Input: part model. Units: mm. Frame: model coordinates. Face numbers are marked on the shaded views. A direction names the side the tool comes from. Give positions to 0.01 mm unless a question says otherwise; leave off trailing zeros. Order: outer loops, then holes, each group sorted by start corner. A loop starts at its lowest first (then second) coordinate and runs counter-clockwise, first axis right, second up. Notation, with made-up numbers: (49.5, -29.75) -> (92.5, -29.75) arc R31 cw to (92.5, 2.25) -> close; hole circle Ø11 at (42, 18.25). An arc over 180 degrees is marked (long way). Use a Markdown table: item, result. Add a question column.
from build123d import *

# Parameters (mm, degrees)
EXTRUDE_1_DEPTH      = 25
CUT_EXTRUDE_4_DEPTH  = 80.457942189
SKETCH_7_W           = 16.60831278
SKETCH_7_H           = 38.473598513
CUT_EXTRUDE_14_DEPTH = 80.457942189
SKETCH_8_W           = 5
SKETCH_8_H           = 30.968526609
EXTRUDE_2_DEPTH      = 25
EXTRUDE_3_DEPTH      = 25
FILLET_2_R           = 3
FILLET_4_R           = 1
SKETCH_10_W          = 2
SKETCH_10_H          = 4
CUT_EXTRUDE_15_DEPTH = 78.792556685
SKETCH_11_W          = 10.357145721
SKETCH_11_H          = 16.019748685
CUT_EXTRUDE_16_DEPTH = 80.457942189


with BuildPart() as part:
    # Эскиз1 → Бобышка-Вытянуть1 (new body)
    with BuildSketch(Plane(origin=(0, 0, 0), x_dir=(1, 0, 0), z_dir=(0, 1, 0))):
        Polygon((-66.825757576, 34.969739794), (-66.825757576, 29.969739794), (-63.825757576, 29.969739794), (-63.825757576, 31.969739794), (-38.825757576, 31.969739794), (-38.825757576, 6.969739794), (-63.825757576, 6.969739794), (-63.825757576, 8.969739794), (-66.825757576, 8.969739794), (-66.825757576, 3.969739794), (-22.123470102, 3.969739794), (-36.579007505, 34.969739794), align=None)
    extrude(amount=EXTRUDE_1_DEPTH)

    # Эскиз3 → Вырез-Вытянуть4 (cut, through all)
    with BuildSketch(Plane.XZ):
        Polygon((-66.825757576, -3.969739794), (-65.325757576, -8.969739794), (-66.825757576, -8.969739794), align=None)
        Polygon((-66.825757576, -29.969739794), (-66.825757576, -34.969739794), (-65.325757576, -29.969739794), align=None)
    extrude(amount=-CUT_EXTRUDE_4_DEPTH, mode=Mode.SUBTRACT)

    # Эскиз7 → Вырез-Вытянуть14 (cut, through all)
    with BuildSketch(Plane(origin=(0, 0, 0), x_dir=(-1, 0, 0), z_dir=(0, -1, 0))):
        with Locations((27.703474463, 20.539743139)):
            Rectangle(SKETCH_7_W, SKETCH_7_H)
    extrude(amount=-CUT_EXTRUDE_14_DEPTH, mode=Mode.SUBTRACT)

    # Эскиз8 → Бобышка-Вытянуть2 (add)
    with BuildSketch(Plane(origin=(0, 0, 0), x_dir=(-1, 0, 0), z_dir=(0, -1, 0))):
        with Locations((36.298943925, 19.454003098)):
            Rectangle(SKETCH_8_W, SKETCH_8_H)
    extrude(amount=-EXTRUDE_2_DEPTH)

    # Эскиз9 → Бобышка-Вытянуть3 (add)
    with BuildSketch(Plane.XZ):
        with BuildLine():
            Line((-25.798943925, -9.121669553), (-24.000865345, -7.695483003))
            ThreePointArc((-24.000865345, -7.695483003), (-36.096342696, -11.954003099), (-24.000865345, -16.212523195))
            Line((-24.000865345, -16.212523195), (-25.798943925, -14.786336644))
            ThreePointArc((-25.798943925, -14.786336644), (-33.80140029, -11.954003099), (-25.798943925, -9.121669553))
        make_face()
        with BuildLine():
            Line((-25.798943925, -24.130682885), (-24.000865345, -22.7126007))
            ThreePointArc((-24.000865345, -22.7126007), (-36.0856317, -26.954003099), (-24.000865345, -31.195405497))
            Line((-24.000865345, -31.195405497), (-25.798943925, -29.777323313))
            ThreePointArc((-25.798943925, -29.777323313), (-33.795735785, -26.954003099), (-25.798943925, -24.130682885))
        make_face()
    extrude(amount=-EXTRUDE_3_DEPTH)

    # Скругление2
    # the kernel refuses this fillet: 3 mm, written as the material it adds along each edge
    with BuildSketch(Plane(origin=(-33.798943925, 25, -6.859434417), x_dir=(0, 0, 1), z_dir=(0, -1, 0))) as fillet_2_piece_1:
        with BuildLine():
            CenterArc((4.502629254, -2.529514158), FILLET_2_R, 122.523458888, 69.079199353)
            Line((1.563931496, -3.132884263), (1.505157541, -3.144951665))
            ThreePointArc((1.505157541, -3.144951665), (0.933475042, -1.490808901), (-0.044969279, -0.039721077))
            Line((-0.044969279, -0.039721077), (0, 0.06))
            ThreePointArc((0, 0.06), (1.444847312, 0.06), (2.85743593, 0.050590283))
            Line((2.85743593, 0.050590283), (2.889694623, 0))
        make_face()
    extrude(amount=25)
    with BuildSketch(Plane(origin=(-33.798943925, 25, -32.034271886), x_dir=(0, 0, -1), z_dir=(0, -1, 0))) as fillet_2_piece_2:
        with BuildLine():
            CenterArc((4.507255062, 2.535656843), FILLET_2_R, 168.421178081, 69.274223823)
            Line((1.568306542, 3.137804332), (1.509527572, 3.149847282))
            ThreePointArc((1.509527572, 3.149847282), (0.936720457, 1.492647534), (-0.044913828, 0.039783766))
            Line((-0.044913828, 0.039783766), (0, -0.06))
            ThreePointArc((0, -0.06), (1.451997259, -0.06), (2.871929307, -0.050713137))
            Line((2.871929307, -0.050713137), (2.903994517, 0))
        make_face()
    extrude(amount=25)

    # Скругление4
    fillet_4_edges = [part.edges().sort_by_distance(p)[0] for p in [
        (-24.000865345, 12.5, -7.695483003),
        (-24.000865345, 12.5, -16.212523195),
        (-24.000865345, 12.5, -22.7126007),
        (-24.000865345, 12.5, -31.195405497),
    ]]
    fillet(fillet_4_edges, radius=FILLET_4_R)

    # Эскиз10 → Вырез-Вытянуть15 (cut, through all)
    with BuildSketch(Plane.XY.offset(-3.969739794)):
        with Locations((-32.798943925, 18)):
            Rectangle(SKETCH_10_W, SKETCH_10_H)
        with Locations((-32.798943925, 7)):
            Rectangle(SKETCH_10_W, SKETCH_10_H)
    extrude(amount=-CUT_EXTRUDE_15_DEPTH, mode=Mode.SUBTRACT)

    # Эскиз11 → Вырез-Вытянуть16 (cut, through all)
    with BuildSketch(Plane.XZ):
        with Locations((-28.620371065, -11.979614137)):
            Rectangle(SKETCH_11_W, SKETCH_11_H)
    extrude(amount=-CUT_EXTRUDE_16_DEPTH, mode=Mode.SUBTRACT)


solid = part.part
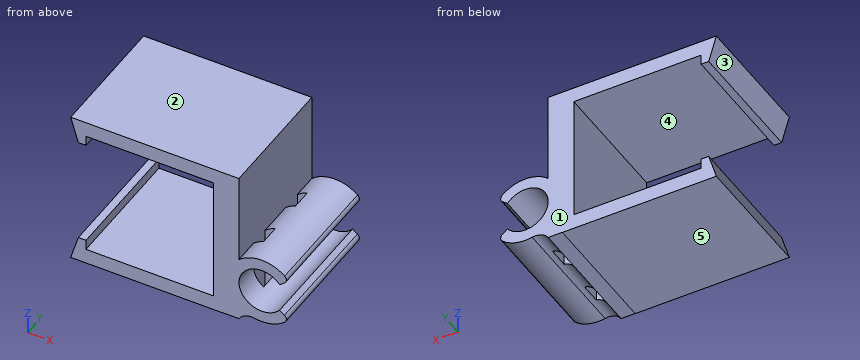
Q1. Ray query, line 1 (Z direction, x = -62, y = 8.75); line 2 (X direction, y = 8, z = -31); line 3 (X direction, y = 3, z = -10). Return the intervals inside material, ascending.
Q2. Section query B-B (y = 6.75). Give the number of separate pieces and of enclosed holes in the cut face, plus the area to 3 significant figures.
Q3. Section query C-C (z = -15). Return loops of the section in (x, y).
Q4. Draft query along Z for the marked faces 1, 2 and 3. Return one class per face: +Z half, -Z half, draft (parallel to the pull), parting line (faces both ways), or undercut.
Q5. Section query A-A (x = -30). Return loops of the section in (y, z), plus the area to 3 significant figures.
Q6. Section query D-D (x = -43.5). Return loops of the section in (y, z), plus the area to 3 significant figures.
Q7. Access query for the marked faces 4 and 5. Directions: +Z, -Z, +X, -X, +Y, -Y. A direction counts if a zero-diameter tool reaches every point of the face in a straight line with its end or side. Return the directions, or none.
Q8. First-contact query: pin 1 (2 mm diameter, centred on x = -35, y = 8, fed in from -Z); pin 2 (1 mm diameter, centred on y = 10, z = -8, fed in from +X); pin 3 (12.5 mm diameter, centred on y = 7, z = -16, fed in from -X). Flat tips, straight axial feed; report the tip coordinate or a pass-through.
Solution:
| question | item | result |
|---|---|---|
| 1 | line 1 | z = -34.97 to -31.97, -6.97 to -3.97 |
| 1 | line 2 | x = -65.63 to -63.83, -38.83 to -33.8, -31.8 to -31.26, -27.34 to -24.53 |
| 1 | line 3 | x = -38.83 to -33.8 |
| 2 | separate pieces | 3 |
| 2 | enclosed holes | 0 |
| 2 | area | 363 mm² |
| 3 | outline | (-38.83, 0) -> (-33.8, 0) -> (-33.8, 25) -> (-38.83, 25) -> close |
| 4 | face 1 | draft |
| 4 | face 2 | +Z half |
| 4 | face 3 | undercut |
| 5 | outline | (0, -33.7) -> (25, -33.7) -> (25, -31.4) -> (0, -31.4) -> close; (0, -22.51) -> (25, -22.51) -> (25, -20.2) -> (0, -20.2) -> close |
| 5 | area | 115 mm² |
| 6 | outline | (0, -34.97) -> (25, -34.97) -> (25, -31.97) -> (0, -31.97) -> close; (0, -6.97) -> (25, -6.97) -> (25, -3.97) -> (0, -3.97) -> close |
| 6 | area | 150 mm² |
| 7 | face 4 | +Y, -Y |
| 7 | face 5 | -Z, +X, -X, +Y, -Y |
| 8 | pin 1 | stops at z = -34.94 |
| 8 | pin 2 | stops at x = -33.8 |
| 8 | pin 3 | stops at x = -38.83 |
